Work out the finished part from the listing and answer in its coordinate system (mm). Round coordinates to 2 decimals unless told otherwise and drop trailing zeros. Order: outer loops, then holes, each group sorted by start corner. A loop starts at its lowest first (then second) coordinate and runs counter-clockwise, first axis right, second up. Notation, with made-up numbers: (-6.75, 14) - (17.25, 14) arc R25 cw to (17.25, 48) - close; hole circle Ø9 at (-18.75, 57). An arc over 180 degrees is marked (long way). Use CSV: the item, a comma, the result in double quotes.
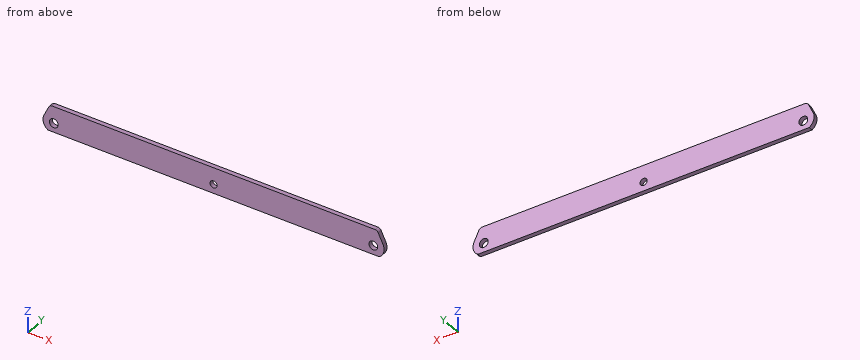
from build123d import *
from build123d import SkipClean  # not in build123d's __all__

# Parameters (mm, degrees)
F0_R     = 5.125
F1_DEPTH = 5


with BuildPart() as f1:
    # F0 (on Front) → F1 (new body)
    with BuildSketch(Plane.XZ):
        with BuildLine():
            Line((-191.7823299831, 0), (0, 0))
            Line((0, 0), (0, 6.375))
            ThreePointArc((0, 6.375), (-4.125, 10.5), (0, 14.625))
            Line((0, 14.625), (0, 30))
            Line((0, 30), (-187, 30))
            ThreePointArc((-187, 30), (-189.1316333954, 29.3846918719), (-190.6074611137, 27.7280695337))
            Line((-190.6074611137, 27.7280695337), (-196.2733159802, 15.9002172929))
            ThreePointArc((-196.2733159802, 15.9002172929), (-197.029373021, 7.1023265723), (-191.7823299831, 0))
        make_face()
        with Locations((-185, 10.5)):
            Circle(F0_R, mode=Mode.SUBTRACT)
    extrude(amount=F1_DEPTH)

    # F2: F1 across plane


with BuildPart() as f1_1:
    add(f1.part, clean=False)
    with SkipClean():  # cleaning this boolean's faces spoils the solid; the shape is the same uncleaned
        add(f1.part.mirror(Plane.YZ), clean=False)


solid = f1_1.part
(1) Find the intervals of material crossed by L1, parallel to X at y = -4.05, z = 11; L2, parallel to Z at x = -185, y = -2.65 (3 decimals); L3, parallel to Z at x = 0, y = -3.9 (3 decimals), in increasing order. Write a range as from..to.
Findings below:
L1,"x = -197.49..-190.1, -179.9..-4.09, 4.09..179.9, 190.1..197.49"
L2,"z = 0..5.375, 15.625..30"
L3,"z = 0..6.375, 14.625..30"
(2) Find section B-B (z = 10.5). Determine the outline of the cut face in (x, y) (3 decimals).
Findings below:
outline,"(-197.5, -5) - (-190.125, -5) - (-190.125, 0) - (-197.5, 0) - close; (-179.875, -5) - (-4.125, -5) - (-4.125, 0) - (-179.875, 0) - close; (4.125, -5) - (179.875, -5) - (179.875, 0) - (4.125, 0) - close; (190.125, -5) - (197.5, -5) - (197.5, 0) - (190.125, 0) - close"
(3) Each of these flat-tipped pins is pushed along its axis until it touches: pin 1 (9 mm diameter, centred on x = 185, z = 10.5, fed in from -Y) (3 decimals); pin 2 (9.5 mm diameter, centred on x = 0, z = 10.5, fed in from +Y). Where does it stop, or does it pass through?
Findings below:
pin 1,"passes through"
pin 2,"stops at y = 0"
(4) Find section A-A (y = -1.7). Determine the outline of the cut face in (x, z) (3 decimals), and give its area (3 significant figures).
Findings below:
outline,"(-196.273, 15.9) arc R12.5 ccw to (-191.782, 0) - (191.782, 0) arc R12.5 ccw to (196.273, 15.9) - (190.607, 27.728) arc R4 ccw to (187, 30) - (-187, 30) arc R4 ccw to (-190.607, 27.728) - close; hole circle Ø10.25 at (-185, 10.5); hole circle Ø8.25 at (0, 10.5); hole circle Ø10.25 at (185, 10.5)"
area,"11,500 mm²"
(5) Find section C-C (x = 0). Determine the outline of the cut face in (y, z) (3 decimals).
Findings below:
outline,"(-5, 0) - (0, 0) - (0, 6.375) - (-5, 6.375) - close; (-5, 14.625) - (0, 14.625) - (0, 30) - (-5, 30) - close"
